Verification items for the finished model (mm, model axes). A direction names the side the tool comes from. Give positions to 0.01 mm unless a question says otherwise; leave off trailing zeros. Write each loop counter-clockwise with the first axis right and the second up, starting at its lowest first coordinate (ties: lowest second). Pieces come first, ordered by that corner, then holes. Notation, with made-up numbers: M 82.25,74 L 108.25,74 A25 ccw 108.25,111 Z; hole C 16,-28.5 d6. An arc over 180 degrees is marked long. Answer as a JSON object with one key per item and string values.
```python
from build123d import *

# Parameters (mm, degrees)
F1_DEPTH = 12.5


# Not quite as in the source:
# - ends of sketch curves that miss each other by under 0.0002 mm in the source are joined


with BuildPart() as f1:
    # F0 (on Top) → F1 (new body, symmetric)
    with BuildSketch(Plane.XY):
        with BuildLine():
            ThreePointArc((14.9995966273, -0.1100046231), (14.9998991565, -0.0550026813), (15, 0))
            ThreePointArc((15, 0), (14.9998991565, 0.0550026813), (14.9995966273, 0.1100046231))
            Line((14.9995966273, 0.1100046231), (13.0450340373, 3.4954063355))
            Line((13.0450340373, 3.4954063355), (13.0450340373, 7.4045315155))
            ThreePointArc((13.0450340373, 7.4045315155), (12.9903810568, 7.5), (12.9350294143, 7.5950651118))
            Line((12.9350294143, 7.5950651118), (9.5496277018, 9.5496277018))
            Line((9.5496277018, 9.5496277018), (7.5950651118, 12.9350294143))
            ThreePointArc((7.5950651118, 12.9350294143), (7.5, 12.9903810568), (7.4045315155, 13.0450340373))
            Line((7.4045315155, 13.0450340373), (3.4954063355, 13.0450340373))
            Line((3.4954063355, 13.0450340373), (0.1100046231, 14.9995966273))
            ThreePointArc((0.1100046231, 14.9995966273), (0, 15), (-0.1100046231, 14.9995966273))
            Line((-0.1100046231, 14.9995966273), (-3.4954063355, 13.0450340373))
            Line((-3.4954063355, 13.0450340373), (-7.4045315155, 13.0450340373))
            ThreePointArc((-7.4045315155, 13.0450340373), (-7.5, 12.9903810568), (-7.5950651118, 12.9350294143))
            Line((-7.5950651118, 12.9350294143), (-9.5496277018, 9.5496277018))
            Line((-9.5496277018, 9.5496277018), (-12.9350294143, 7.5950651118))
            ThreePointArc((-12.9350294143, 7.5950651118), (-12.9903810568, 7.5), (-13.0450340373, 7.4045315155))
            Line((-13.0450340373, 7.4045315155), (-13.0450340373, 6))
            Line((-13.0450340373, 6), (-8, 6))
            ThreePointArc((-8, 6), (3.1622775895, 9.4868327685), (9.9999997765, 0))
            ThreePointArc((9.9999997765, 0), (3.1622775895, -9.4868327685), (-7.9999998212, -5.9999998659))
            Line((-7.9999998212, -5.9999998659), (-13.0450340373, -6))
            Line((-13.0450340373, -6), (-13.0450340373, -7.4045315155))
            ThreePointArc((-13.0450340373, -7.4045315155), (-12.9903810568, -7.5), (-12.9350294143, -7.5950651118))
            Line((-12.9350294143, -7.5950651118), (-9.5496277018, -9.5496277018))
            Line((-9.5496277018, -9.5496277018), (-7.5950651118, -12.9350294143))
            ThreePointArc((-7.5950651118, -12.9350294143), (-7.5, -12.9903810568), (-7.4045315155, -13.0450340373))
            Line((-7.4045315155, -13.0450340373), (-3.4954063355, -13.0450340373))
            Line((-3.4954063355, -13.0450340373), (-0.1100046231, -14.9995966273))
            ThreePointArc((-0.1100046231, -14.9995966273), (0, -15), (0.1100046231, -14.9995966273))
            Line((0.1100046231, -14.9995966273), (3.4954063355, -13.0450340373))
            Line((3.4954063355, -13.0450340373), (7.4045315155, -13.0450340373))
            ThreePointArc((7.4045315155, -13.0450340373), (7.5, -12.9903810568), (7.5950651118, -12.9350294143))
            Line((7.5950651118, -12.9350294143), (9.5496277018, -9.5496277018))
            Line((9.5496277018, -9.5496277018), (12.9350294143, -7.5950651118))
            ThreePointArc((12.9350294143, -7.5950651118), (12.9903810568, -7.5), (13.0450340373, -7.4045315155))
            Line((13.0450340373, -7.4045315155), (13.0450340373, -3.4954063355))
            Line((13.0450340373, -3.4954063355), (14.9995966273, -0.1100046231))
        make_face()
    extrude(amount=F1_DEPTH, both=True)


solid = f1.part
```
1) Section check C-C on y = 2.5. Record the boundary of the cut face in (x, z).
Completed:
{"outline": "M 9.68,-12.5 L 13.62,-12.5 L 13.62,12.5 L 9.68,12.5 Z"}
2) Access from +Z, -Z, +X, -X, +Y, -Y to the whole of each face (thin tool, end or side, straight path). Record for faces 1 (the face through (-10, -6, 0)), 2 (the face through (5, 13.045, 0)), 3 (the face through (5, -13.045, 0)).
Completed:
{"face 1": "+Z, -Z, -X", "face 2": "+Z, -Z, +X, +Y", "face 3": "+Z, -Z, +X, -Y"}
3) Section check D-D on y = -5.5. Record the boundary of the cut face in (x, z), and give its area (3 significant figures).
Completed:
{"outline": "M 8.35,-12.5 L 13.05,-12.5 L 13.05,12.5 L 8.35,12.5 Z", "area": "117 mm2"}
4) Go/stop test with flat-tipped pins: pin 1 (8 mm diameter, centred on x = 10.5, y = -10, fed in from +Z); pin 2 (2 mm diameter, centred on x = -4, z = 7.5, fed in from +Y); pin 3 (1.5 mm diameter, centred on x = -1.5, z = -4.5, fed in from +Y); pin 4 (5.5 mm diameter, centred on x = -10, z = 1, fed in from +Y). Record where each tip stops, or that it passes through.
Completed:
{"pin 1": "stops at z = 12.5", "pin 2": "stops at y = 13.33", "pin 3": "stops at y = 14.63", "pin 4": "stops at y = 13.05"}
5) Section check B-B on y = 6.5. Record the boundary of the cut face in (x, z), and give its area (3 significant figures).
Completed:
{"outline": "M -13.05,-12.5 L -7.6,-12.5 L -7.6,12.5 L -13.05,12.5 Z; M 7.6,-12.5 L 13.05,-12.5 L 13.05,12.5 L 7.6,12.5 Z", "area": "272 mm2"}
6) Section check A-A on x = 1. Record the boundary of the cut face in (y, z).
Completed:
{"outline": "M -14.49,-12.5 L -9.95,-12.5 L -9.95,12.5 L -14.49,12.5 Z; M 9.95,-12.5 L 14.49,-12.5 L 14.49,12.5 L 9.95,12.5 Z"}
7) Release check for a two-part mould opening along Y. For faces 4 (the face through (-11, 6, 0)), 5 (the face through (-5, 13.045, 0)), 6 (the face through (-1.826, -14.009, 0.175)) record: pulls with the +Y half, pulls with the -Y half, needs draft (parallel to the pull), parting line crosses it, or undercut.
Completed:
{"face 4": "undercut", "face 5": "pulls with the +Y half", "face 6": "pulls with the -Y half"}
8) Thickness scan on L1, parallel to Y at x = 6.5, z = 2.25; L2, parallel to Y at x = 9, z = 6.5; L3, parallel to X at y = 10.5, z = 5.5. Record the ranges inside material, lowest first.
Completed:
{"L1": "y = -13.05 to -7.6, 7.6 to 13.05", "L2": "y = -10.5 to -4.36, 4.36 to 10.5", "L3": "x = -9 to 9"}
